Autodesk Inventor part; units mm, degrees
ref_plane "YZ Plane" through (0, 0, 0) normal (1, 0, 0) x (0, 1, 0)
ref_plane "XZ Plane" through (0, 0, 0) normal (0, 1, 0) x (-1, 0, 0)
ref_plane "XY Plane" through (0, 0, 0) normal (0, 0, 1) x (1, 0, 0)
sketch "Sketch1" plane through (0, 0, 0) normal (0, 1, 0) x (-1, 0, 0)
  circle A0 centre (0, 0) radius 34
  circle A1 centre (9.5, 0) radius 1.6
  circle A2 centre (4.75, 8.2272) radius 1.6
  circle A3 centre (-4.75, 8.2272) radius 1.6
  circle A4 centre (-9.5, 0) radius 1.6
  circle A5 centre (-4.75, -8.2272) radius 1.6
  circle A6 centre (4.75, -8.2272) radius 1.6
  circle A7 centre (30, 0) radius 1.175
  circle A8 centre (21.2132, 21.2132) radius 1.175
  circle A9 centre (0, 30) radius 1.175
  circle A10 centre (-21.2132, 21.2132) radius 1.175
  circle A11 centre (-30, 0) radius 1.175
  circle A12 centre (-21.2132, -21.2132) radius 1.175
  circle A13 centre (0, -30) radius 1.175
  circle A14 centre (21.2132, -21.2132) radius 1.175
  dimension "d0" = 68
  dimension "d1" = 3.2
  dimension "d2" = 9.5
  dimension "d3" = 0
  dimension "d6" = 360
  dimension "d10" = 2.35
  dimension "d11" = 0
  dimension "d12" = 30
  dimension "d15" = 360
extrude "Extrusion3" add sketch "Sketch1" along normal blind 5
sketch "Sketch5" plane through (0, 0, 0) normal (0, -1, 0) x (1, 0, 0)
  circle A0 centre (0, 0) radius 34
  circle A1 centre (21.2132, 21.2132) radius 1.175
  circle A2 centre (30, 0) radius 1.175
  circle A3 centre (21.2132, -21.2132) radius 1.175
  circle A4 centre (0, -30) radius 1.175
  circle A5 centre (-21.2132, -21.2132) radius 1.175
  circle A6 centre (-30, 0) radius 1.175
  circle A7 centre (-21.2132, 21.2132) radius 1.175
  circle A8 centre (0, 30) radius 1.175
  circle A9 centre (0, 0) radius 27.25
  circle A10 centre (21.2132, 21.2132) radius 1.175
  circle A11 centre (30, 0) radius 1.175
  circle A12 centre (21.2132, -21.2132) radius 1.175
  circle A13 centre (0, -30) radius 1.175
  circle A14 centre (-21.2132, -21.2132) radius 1.175
  circle A15 centre (-30, 0) radius 1.175
  circle A16 centre (-21.2132, 21.2132) radius 1.175
  circle A17 centre (0, 30) radius 1.175
  circle A18 centre (0, 30) radius 1.225
  circle A19 centre (0, 0) radius 34
  dimension "d21" = 54.5
extrude "Extrusion4" add sketch "Sketch5" along normal blind 26.68 contours A0 | A18
sketch "Sketch6" plane through (0, 5, 0) normal (0, 1, 0) x (1, 0, 0)
  circle A0 centre (0, 0) radius 34
extrude "Extrusion5" cut sketch "Sketch6" against normal blind 5
properties part number "sprocketsHolder" material "ABS Plastic"
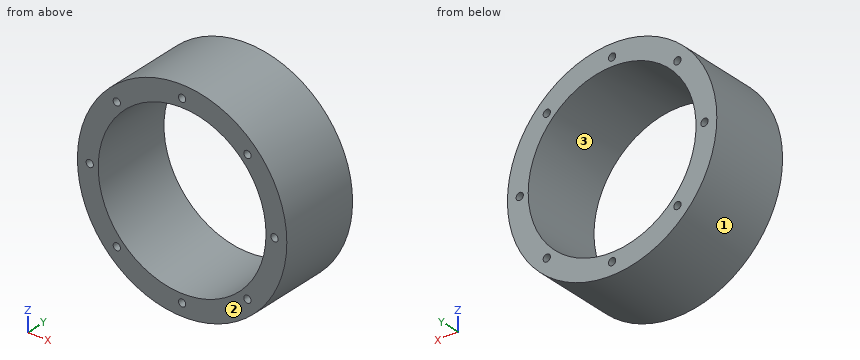
Can you work these out from the model? Positions are in its coordinate system, mm. Face numbers are marked on the shaded views. Round coordinates to 2 decimals unless told otherwise and drop trailing zeros. Order: outer loops, then holes, each group sorted by start corner. A loop starts at its lowest first (then second) coordinate and runs counter-clockwise, first axis right, second up. Notation, with made-up numbers: (49.5, -11.5) -> (93.5, -11.5) arc R35 ccw to (93.5, 26.5) -> close; hole circle Ø9 at (77, -38.75). An arc over 180 degrees is marked (long way). Return JSON: item names as keys, results as strings. Group by question number.
1. We'd pull the mould along X, two halves only. Please class the marked faces 1, 2 and 3: released by +X, released by -X, zero draft, split by the parting line, or undercut.
2. I need wall thicknesses on line 1 (Z direction, x = 0, y = -10.5) (3 decimals); line 2 (X direction, y = -24.75, z = 21.5); line 3 (Z direction, x = 3, y = -4.5). Which ranges of each line are inside material? Lowest first, please. Write a range as [from, to].
3. Will these pins go through, and if not, where does the flat tip stop? pin 1 (3 mm diameter, centred on y = -3.5, z = -26.5, fed in from +X); pin 2 (5 mm diameter, centred on y = -15.5, z = -11, fed in from -X); pin 3 (5 mm diameter, centred on y = -12, z = 19, fed in from -X).
4. If we section it at A-A, the plane z = -30: Write out the boundary of the cut face in (x, y) (3 decimals), then the cut area to 3 significant figures.
5. If we section it at B-B, the plane x = 30: Write out the boundary of the cut face in (y, z) (3 decimals), then the cut area to 3 significant figures.
6. If we section it at C-C, the plane y = -24.5: Count the separate pieces of the cut face and the enclosed holes in it, then the cut area to 3 significant figures.
Output values:
{
 "1": {"face 1": "split by the parting line", "face 2": "zero draft", "face 3": "undercut"},
 "2": {"line 1": "[-34, -31.175], [-28.825, -27.25], [27.25, 28.825], [31.175, 34]", "line 2": "[-26.34, -22.35], [-20.07, -16.74], [16.74, 20.07], [22.35, 26.34]", "line 3": "[-33.87, -27.08], [27.08, 33.87]"},
 "3": {"pin 1": "x = 23.04", "pin 2": "x = -32.92", "pin 3": "x = -29.73"},
 "4": {"outline": "(-16, -26.68) -> (-1.175, -26.68) -> (-1.175, 0) -> (-16, 0) -> close; (1.175, -26.68) -> (16, -26.68) -> (16, 0) -> (1.175, 0) -> close", "area": "791 mm²"},
 "5": {"outline": "(-26.68, -16) -> (0, -16) -> (0, -1.175) -> (-26.68, -1.175) -> close; (-26.68, 1.175) -> (0, 1.175) -> (0, 16) -> (-26.68, 16) -> close", "area": "791 mm²"},
 "6": {"separate pieces": "1", "enclosed holes": "9", "area": "1,260 mm²"}
}
